Check sheet for the modelled part. Datum: model origin and axes. Units: mm. Give positions to 0.01 mm unless a question says otherwise; leave off trailing zeros. Loops run counter-clockwise (first coordinate to the right, second up) from the corner with the lowest first, then second, coordinate; pieces in that order, holes last. Notation, with made-up numbers: (3, 22) -> (62, 22) arc R20 ccw to (62, 38) -> close; hole circle Ø9 at (-5.75, 22.5). An arc over 180 degrees is marked (long way). Write each question's results on one line, items separated by ' | '. Start each with the question number.
1. Cross-section at B-B on x = 20. Record the boundary of the cut face in (y, z), and give its area (3 significant figures).
2. Material ranges on L1, parallel to Y at x = -0.75, z = 264.5; L2, parallel to X at y = 84.75, z = 203, recorded low to high. Write a range as from..to.
3. Cross-section at C-C on z = 386. Record the boundary of the cut face in (x, y).
4. Cross-section at A-A on y = 87.25. Record the boundary of the cut face in (x, z).
from build123d import *

# Parameters (mm, degrees)
ESBO_O1_W                = 30
ESBO_O1_H                = 30
RESSALTO_EXTRUS_O1_DEPTH = 440
CASCA1_T                 = -2


with BuildPart() as part:
    # Esboço1 → Ressalto-extrusão1 (new body)
    with BuildSketch(Plane.XY):
        with Locations((10.655165912, 87.212171493)):
            Rectangle(ESBO_O1_W, ESBO_O1_H)
    extrude(amount=RESSALTO_EXTRUS_O1_DEPTH)

    # Casca1
    casca1_openings = [part.faces().sort_by_distance(p)[0] for p in [
        (10.655165912, 87.212171493, 440),
        (10.655165912, 87.212171493, 0),
    ]]
    offset(amount=CASCA1_T, openings=casca1_openings, kind=Kind.INTERSECTION)


solid = part.part
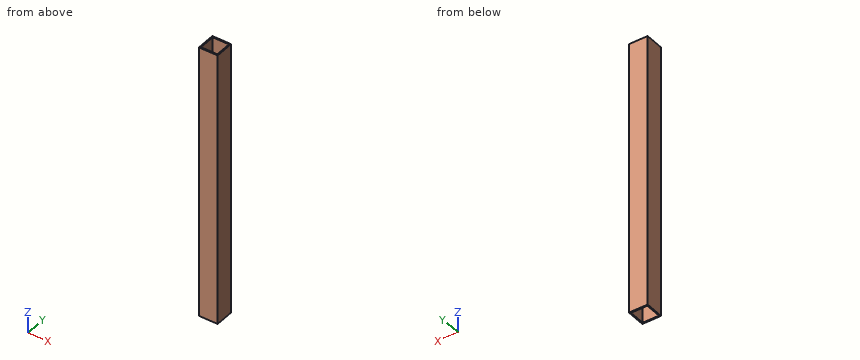
Geometry says:
1) outline: (72.21, 0) -> (74.21, 0) -> (74.21, 440) -> (72.21, 440) -> close; (100.21, 0) -> (102.21, 0) -> (102.21, 440) -> (100.21, 440) -> close | area: 1,760 mm^2
2) L1: 72.21..74.21, 100.21..102.21 | L2: -4.34..-2.34, 23.66..25.66
3) outline: (-4.34, 72.21) -> (25.66, 72.21) -> (25.66, 102.21) -> (-4.34, 102.21) -> close; hole (-2.34, 74.21) -> (23.66, 74.21) -> (23.66, 100.21) -> (-2.34, 100.21) -> close
4) outline: (-4.34, 0) -> (-2.34, 0) -> (-2.34, 440) -> (-4.34, 440) -> close; (23.66, 0) -> (25.66, 0) -> (25.66, 440) -> (23.66, 440) -> close
